Read the model definition and answer for the solid it produces. Units are mm, in the model's axes. A direction names the side the tool comes from. Round coordinates to 2 decimals unless told otherwise and drop trailing zeros. Write each loop counter-clockwise with the first axis right and the second up, starting at its lowest first coordinate (ties: lowest second). Pieces come first, ordered by that corner, then holes. Notation, with made-up numbers: (61.5, -32) - (76.5, -32) arc R36 cw to (76.5, 6) - close; hole circle Ø8 at (13, -33). An arc over 180 degrees is marked (long way). One line per item, written item: value. Start each with the question number.
(1) A flat-ended cylindrical pin translates along its axis: pin 1 Ø1.5 at (x, y) = (-60.5, 36) entering from +Z. Find the tip coordinate at first contact, or state that the pin passes through.
(2) A cutting plane is placed at A-A, the plane z = 32. Determine the outline of the cut face in (x, y), plus the area to 3 significant figures.
(3) The mould has two halves that part along Y. Classify faces 1 (the face through (-67.14, -62.43, 18.78)), 2 (the face through (-68.949, -4, 19)), 3 (the face through (-63.602, -4, 25)): +Y half, -Y half, draft (parallel to the pull), parting line (faces both ways), or undercut.
(4) Find the intervals of material crossed by L1, parallel to Y at x = -21, z = 13; L2, parallel to X at y = -53, z = 13; L3, parallel to Z at x = -23, y = 12, in increasing order.
(5) For faces 4 (the face through (-37, 51.066, 25)), 5 (the face through (-65, -4, 38.1)), determine the directions among +Z, -Z, +X, -X, +Y, -Y from which every point of the face is accessible in a straight line to the end or side of a thin tool.
(6) A cutting plane is placed at C-C, the plane x = -20. Determine the outline of the cut face in (y, z), plus the area to 3 significant figures.
(7) A cutting plane is placed at B-B, the plane y = -50.5. Determine the outline of the cut face in (x, z), plus the area to 3 significant figures.
from build123d import *

# Parameters (mm, degrees)
F0_W     = 58.993546
F0_H     = 109.506775
F1_DEPTH = 38.1
F2_DEPTH = 12.7
F3_R     = 5.08


with BuildPart() as f1:
    # F0 (on Top) → F1 (new body)
    with BuildSketch(Plane.XY):
        with BuildLine():
            Line((-62.598708, -64.339839), (-6.35, -64.339839))
            ThreePointArc((-6.35, -64.339839), (-1.859872, -62.479967), (0, -57.989839))
            Line((0, -57.989839), (0, 49.140807))
            ThreePointArc((0, 49.140807), (-1.859872, 53.630935), (-6.35, 55.490807))
            Line((-6.35, 55.490807), (-62.598708, 55.490807))
            ThreePointArc((-62.598708, 55.490807), (-67.088837, 53.630935), (-68.948708, 49.140807))
            Line((-68.948708, 49.140807), (-68.948708, -57.989839))
            ThreePointArc((-68.948708, -57.989839), (-67.088837, -62.479967), (-62.598708, -64.339839))
        make_face()
        with Locations((-34.105645, -3.687096)):
            Rectangle(F0_W, F0_H, mode=Mode.SUBTRACT)
    extrude(amount=F1_DEPTH)

    # F0 (on Top) → F2 (join)
    with BuildSketch(Plane.XY):
        with Locations((-34.105645, -3.687096)):
            Rectangle(F0_W, F0_H)
    extrude(amount=F2_DEPTH)

    # F3
    f3_edges = [f1.edges().sort_by_distance(p)[0] for p in [
        (-4.608872, 51.066291, 25.4),
    ]]
    fillet(f3_edges, radius=F3_R)


solid = f1.part
Here are the results:
1. pin 1: z = 12.7
2. outline: (-68.95, -57.99) arc R6.35 ccw to (-62.6, -64.34) - (-6.35, -64.34) arc R6.35 ccw to (0, -57.99) - (0, 49.14) arc R6.35 ccw to (-6.35, 55.49) - (-62.6, 55.49) arc R6.35 ccw to (-68.95, 49.14) - close; hole (-63.6, -58.44) - (-4.61, -58.44) - (-4.61, 45.99) arc R5.08 ccw to (-9.69, 51.07) - (-63.6, 51.07) - close
2. area: 1,770 mm²
3. face 1: -Y half
3. face 2: draft
3. face 3: undercut
4. L1: -64.34 to -58.44, 51.07 to 55.49
4. L2: -68.95 to -63.6, -4.61 to 0
4. L3: 0 to 12.7
5. face 4: +Z
5. face 5: +Z, +X, -X, +Y, -Y
6. outline: (-64.34, 0) - (55.49, 0) - (55.49, 38.1) - (51.07, 38.1) - (51.07, 12.7) - (-58.44, 12.7) - (-58.44, 38.1) - (-64.34, 38.1) - close
6. area: 1,780 mm²
7. outline: (-68.95, 0) - (0, 0) - (0, 38.1) - (-4.61, 38.1) - (-4.61, 12.7) - (-63.6, 12.7) - (-63.6, 38.1) - (-68.95, 38.1) - close
7. area: 1,130 mm²
